```python
from build123d import *

# Parameters (mm, degrees)
BOSS_EXTRUDE1_DEPTH            = 10
BOSS_EXTRUDE1_DEPTH_BACK       = 10
BOSS_EXTRUDE2_START            = -8.5
BOSS_EXTRUDE2_DEPTH            = 17
M4_CLEARANCE_HOLE1_D           = 4.3
M4_CLEARANCE_HOLE1_CSINK_D     = 4.35
M4_CLEARANCE_HOLE1_CSINK_ANGLE = 90
M4_CLEARANCE_HOLE2_D           = 4.3
M4_CLEARANCE_HOLE2_CSINK_D     = 4.35
M4_CLEARANCE_HOLE2_CSINK_ANGLE = 90
CUT_EXTRUDE1_DEPTH             = 89.78154726
CUT_EXTRUDE1_DEPTH_BACK        = 89.78154726


with BuildPart() as part:
    # Sketch2 → Boss-Extrude1 (new, two sides: drawn at the far end of the back side and taken through both)
    with BuildSketch(Plane(origin=(0, 0, 0), x_dir=(0, 0, -1), z_dir=(1, 0, 0)).offset(-BOSS_EXTRUDE1_DEPTH_BACK)):
        with BuildLine():
            Line((0, 13.70642245), (-6, 13.70642245))
            Line((-6, 13.70642245), (-23, 13.70642245))
            Line((-23, 13.70642245), (-78.775396858, 13.70642245))
            Line((-78.775396858, 13.70642245), (-78.775396858, 0))
            ThreePointArc((-78.775396858, 0), (-59.416347042, -5.45481476), (-39.387698429, -7.29357755))
            ThreePointArc((-39.387698429, -7.29357755), (-19.359049816, -5.45481476), (0, 0))
            Line((0, 0), (0, 13.70642245))
        make_face()
    extrude(amount=BOSS_EXTRUDE1_DEPTH + BOSS_EXTRUDE1_DEPTH_BACK)

    # Sketch2<3> → Boss-Extrude2 (add)
    with BuildSketch(Plane(origin=(0, 0, 0), x_dir=(0, 0, -1), z_dir=(1, 0, 0)).offset(BOSS_EXTRUDE2_START)):
        with BuildLine():
            Line((-23, 13.70642245), (-6, 13.70642245))
            Line((-6, 13.70642245), (-6, 35.706422449))
            ThreePointArc((-6, 35.706422449), (-7.171572875, 38.534849574), (-10, 39.706422449))
            Line((-10, 39.706422449), (-19, 39.706422449))
            ThreePointArc((-19, 39.706422449), (-21.828427125, 38.534849574), (-23, 35.706422449))
            Line((-23, 35.706422449), (-23, 28.706422449))
            Line((-23, 28.706422449), (-23, 23.70642245))
            Line((-23, 23.70642245), (-23, 16.70642245))
            Line((-23, 16.70642245), (-23, 13.70642245))
        make_face()
    extrude(amount=BOSS_EXTRUDE2_DEPTH)

    # M4 Clearance Hole1 (through all)
    with Locations(Plane.ZY.offset(8.5)):
        with Locations((10, 32.206422449), (19, 20.20642245)):
            CounterSinkHole(M4_CLEARANCE_HOLE1_D / 2, M4_CLEARANCE_HOLE1_CSINK_D / 2, counter_sink_angle=M4_CLEARANCE_HOLE1_CSINK_ANGLE)

    # M4 Clearance Hole2 (through all)
    with Locations(Plane(origin=(8.5, 0, 0), x_dir=(0, 0, -1), z_dir=(1, 0, 0))):
        with Locations((-19, 32.206422449), (-10, 20.20642245)):
            CounterSinkHole(M4_CLEARANCE_HOLE2_D / 2, M4_CLEARANCE_HOLE2_CSINK_D / 2, counter_sink_angle=M4_CLEARANCE_HOLE2_CSINK_ANGLE)

    # Sketch8 → Cut-Extrude1 (cut, two sides: drawn at the far end of the back side and taken through both)
    with BuildSketch(Plane(origin=(0, 0, 0), x_dir=(0, 0, -1), z_dir=(1, 0, 0)).offset(-CUT_EXTRUDE1_DEPTH_BACK)):
        with BuildLine():
            Line((-5, 3.497117459), (-5, 8.70642245))
            Line((-5, 8.70642245), (-6, 8.70642245))
            Line((-6, 8.70642245), (-23, 8.70642245))
            Line((-23, 8.70642245), (-25.432523452, 8.70642245))
            Line((-25.432523452, 8.70642245), (-12.989242433, 1.079056445))
            ThreePointArc((-12.989242433, 1.079056445), (-8.970583227, 2.208665745), (-5, 3.497117459))
        make_face()
        with BuildLine():
            ThreePointArc((-39.387698429, -2.29357755), (-29.651907949, -1.841243156), (-20, -0.48813724))
            Line((-20, -0.48813724), (-35, 8.70642245))
            Line((-35, 8.70642245), (-50, -1.755910739))
            ThreePointArc((-50, -1.755910739), (-44.700655003, -2.1590747), (-39.387698429, -2.29357755))
        make_face()
        with BuildLine():
            Line((-57.303381238, -0.753851614), (-43.740048051, 8.70642245))
            Line((-43.740048051, 8.70642245), (-73.775396858, 8.70642245))
            Line((-73.775396858, 8.70642245), (-73.775396858, 3.497117459))
            ThreePointArc((-73.775396858, 3.497117459), (-65.625621494, 1.037492126), (-57.303381238, -0.753851614))
        make_face()
    extrude(amount=CUT_EXTRUDE1_DEPTH + CUT_EXTRUDE1_DEPTH_BACK, mode=Mode.SUBTRACT)


solid = part.part
```
Geometry: final body of the model. Coordinates: model frame, mm. A direction names the side the tool comes from. Coordinates: 2 decimals unless noted, no trailing zeros. Order: outer loops, then holes, each group sorted by start corner. A loop starts at its lowest first (then second) coordinate and runs counter-clockwise, first axis right, second up. Notation, with made-up numbers: (87.5, -19.5) - (124.5, -19.5) arc R15 cw to (124.5, 8.5) - close; hole circle Ø3 at (42, 71.5). An arc over 180 degrees is marked (long way). Return JSON: item names as keys, results as strings. Group by question number.
1. Pull-direction query (Z, two-part tool) for faces 1 (the face through (0.131, 34.019, 8.844)), 2 (the face through (0, 25, 6)), 3 (the face through (-10, 6, 40)), 4 (the face through (0, 25, 23)); classes: pulls with the +Z half, pulls with the -Z half, needs draft (parallel to the pull), parting line crosses it, or undercut.
2. Cut plane B-B (y = 5). Output: boundary loops of the cut face in (x, z).
3. Cut plane C-C (x = -5.5). Output: boundary loops of the cut face in (y, z).
4. Cut plane A-A (z = 54.5). Output: boundary loops of the cut face in (x, y).
5. Set-up query: faces 5 (the face through (-0.14, 3.548, 42.395)), 6 (the face through (-8.5, 27, 15)), 7 (the face through (8.5, 27, 15)). Return all of +Z, -Z, +X, -X, +Y, -Y with unobstructed straight access to the full face (end or side cutting, diameter ignored); none if empty.
6. Pin query (flat end, axial travel): pin 1 (5 mm diameter, centred on y = 33, z = 16, fed in from -X); pin 2 (10 mm diameter, centred on x = -5, z = 62, fed in from -Y); pin 3 (5 mm diameter, centred on x = -1.5, y = 21.5, fed in from -Z). Return the tip coordinate at first contact, or that it passes through.
7. Material intervals for line 1 along Y through (x, z) = (2.25, 10); line 2 along Y through (x, z) = (-5.25, 22); line 3 along Z through (x, y) = (7.75, 14), sorted ascending. Write a range as [from, to].
8. Cut plane D-D (y = 16). Output: boundary loops of the cut face in (x, z).
Resolved:
{
 "1": {"face 1": "undercut", "face 2": "pulls with the -Z half", "face 3": "needs draft", "face 4": "pulls with the +Z half"},
 "2": {"outline": "(-10, 0) - (10, 0) - (10, 5) - (-10, 5) - close; (-10, 19.39) - (10, 19.39) - (10, 28.95) - (-10, 28.95) - close; (-10, 40.31) - (10, 40.31) - (10, 49.05) - (-10, 49.05) - close; (-10, 73.78) - (10, 73.78) - (10, 78.78) - (-10, 78.78) - close"},
 "3": {"outline": "(0, 0) - (13.71, 0) - (13.71, 6) - (35.71, 6) arc R4 ccw to (39.71, 10) - (39.71, 19) arc R4 ccw to (35.71, 23) - (13.71, 23) - (13.71, 78.78) - (0, 78.78) arc R110 ccw to start; hole (-1.76, 50) arc R105 ccw to (-0.49, 20) - (8.71, 35) - close; hole (-0.75, 57.3) - (8.71, 43.74) - (8.71, 73.78) - (3.5, 73.78) arc R105 ccw to start; hole (1.08, 12.99) arc R105 ccw to (3.5, 5) - (8.71, 5) - (8.71, 25.43) - close; hole circle Ø4.3 at (20.21, 10); hole circle Ø4.3 at (20.21, 19); hole circle Ø4.3 at (32.21, 10); hole circle Ø4.3 at (32.21, 19)"},
 "4": {"outline": "(-10, -6.25) - (10, -6.25) - (10, 1.2) - (-10, 1.2) - close; (-10, 8.71) - (10, 8.71) - (10, 13.71) - (-10, 13.71) - close"},
 "5": {"face 5": "+X, -X", "face 6": "+Z, -Z, -X, +Y", "face 7": "+Z, -Z, +X, +Y"},
 "6": {"pin 1": "stops at x = -8.5", "pin 2": "stops at y = -5.87", "pin 3": "stops at z = 6"},
 "7": {"line 1": "y = [-3.3, 1.9], [8.71, 18.06], [22.36, 30.06], [34.36, 39.71]", "line 2": "y = [-5.91, -0.84], [0.74, 6.6], [8.71, 38.35]", "line 3": "z = [6, 23]"},
 "8": {"outline": "(-8.5, 6) - (8.5, 6) - (8.5, 23) - (-8.5, 23) - close"}
}
